Geometry: final body of the model. Coordinates: model frame, mm. Face numbers are marked on the shaded views. A direction names the side the tool comes from. Round coordinates to 2 decimals unless told otherwise and drop trailing zeros. Loops run counter-clockwise (first coordinate to the right, second up) from the corner with the lowest first, then second, coordinate; pieces in that order, holes last. Notation, with made-up numbers: M -25,-23 L 4,-23 A20 cw 4,-5 Z; hole C 24,69 d10. An arc over 180 degrees is marked long. Answer as a JSON object with one key per item and string values.
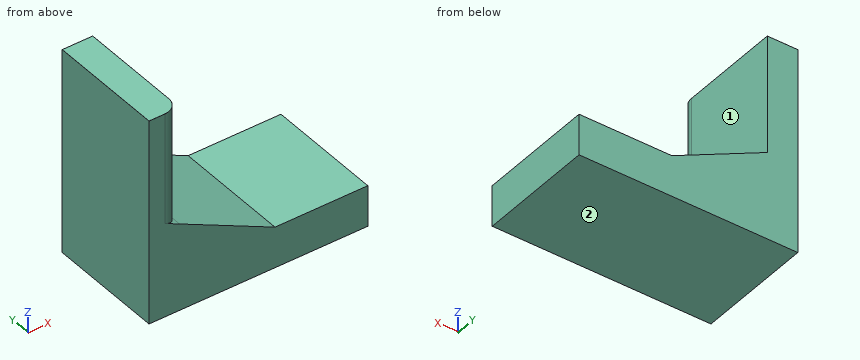
from build123d import *

# Parameters (mm, degrees)
F1_DEPTH    = 40
F2_R        = 0.0241421356
F3_T2_ANGLE = 90
F3_T6_DEPTH = 52.5499999523


# Not quite as in the source:
# - a fillet or chamfer that OpenCascade refuses, or shapes differently, is made with other operations: its cross-section is extruded or revolved along the edge and cut away or added


with BuildPart() as f1:
    # F0 (on Front) → F1 (new body)
    with BuildSketch(Plane.XZ):
        Polygon((0, 40.0499999523), (0, 0), (0, -29.6999998391), (74.2500051856, -29.6999998391), (74.2500051856, -15.7500002533), (42.7500009537, -15.7500002533), (10.349996388, 0), (10.349996388, 40.0499999523), align=None)
    extrude(amount=F1_DEPTH)

    # F2
    f2_edges = [f1.edges().sort_by_distance(p)[0] for p in [
        (10.349996, -20, 40.05),
        (0, -20, 40.05),
        (5.174998, 0, 40.05),
        (5.174998, -40, 40.05),
    ]]
    fillet(f2_edges, radius=F2_R)

    # F3: fillet of radius 5 on 5 edges, made by hand

    # F3_s1 → F3_t2 (revolve, cut)
    with BuildSketch(Plane.YZ.offset(5.349996388)):
        with BuildLine():
            ThreePointArc((-39.9758578644, 40.0499999523), (-39.9929289322, 40.0429288845), (-40, 40.0258578167))
            Line((-40, 40.0258578167), (-40, 40.0499999523))
            Line((-40, 40.0499999523), (-39.9758578644, 40.0499999523))
        make_face()
    revolve(axis=Axis((5.349996388, -35, 40.0499999523), (0, 0, 1)), revolution_arc=F3_T2_ANGLE, mode=Mode.SUBTRACT)


with BuildPart() as f3_tool4:
    # F3_s5 → F3_t6 (new body)
    with BuildSketch(Plane.XY.offset(-12.5)):
        with BuildLine():
            ThreePointArc((10.349996388, -35), (8.8855302939, -38.5355339059), (5.349996388, -40))
            Line((5.349996388, -40), (10.349996388, -40))
            Line((10.349996388, -40), (10.349996388, -35))
        make_face()
    extrude(amount=F3_T6_DEPTH)

    split(bisect_by=Plane(origin=(1.9782716516, 0, 4.0695879055), x_dir=(0, 1, 0), z_dir=(0.4371926627, 0, 0.8993678756)), keep=Keep.TOP)


with BuildPart() as f1_1:
    add(f1.part)

    # F3_t3: cut F3_tool4
    add(f3_tool4.part, mode=Mode.SUBTRACT)


solid = f1_1.part
1) Pin query (flat end, axial travel): P1, Ø16, axis at x = 62.5, y = -25.5, coming from the +Z side. Return the tip coordinate at first contact, or that it passes through.
Results:
{"P1": "z = -15.75"}
2) Section query D-D (z = 1). Return the cut outline in (x, y).
Results:
{"outline": "M 0,-40 L 8.29,-40 L 8.29,-39.04 A5 ccw 10.35,-35 L 10.35,0 L 0,0 Z"}
3) Section query C-C (x = 63.5). Return the cut outline in (y, z), and give its area (3 significant figures).
Results:
{"outline": "M -40,-29.7 L 0,-29.7 L 0,-15.75 L -40,-15.75 Z", "area": "558 mm2"}
4) Reachability of the marked faces 1 and 2 from +Z, -Z, +X, -X, +Y, -Y: full face, straight path, thin tool, end or side. Return the list, or none.
Results:
{"face 1": "+Z, +X, +Y, -Y", "face 2": "-Z, +X, -X, +Y, -Y"}
5) Section query B-B (z = 11). Return the cut outline in (x, y), and give its area (3 significant figures).
Results:
{"outline": "M 0,-40 L 5.35,-40 A5 ccw 10.35,-35 L 10.35,0 L 0,0 Z", "area": "409 mm2"}
6) Ray query, line 1 (X direction, y = -3.5, z = 16.5); line 2 (Z direction, x = 51, y = -36); line 3 (X direction, y = -7, z = -6.5). Return the intervals inside material, ascending.
Results:
{"line 1": "0 to 10.35", "line 2": "-29.7 to -15.75", "line 3": "0 to 23.72"}
